Read the model definition and answer for the solid it produces. Units are mm, in the model's axes. A direction names the side the tool comes from. Coordinates: 2 decimals unless noted, no trailing zeros. Write each loop counter-clockwise with the first axis right and the second up, starting at its lowest first coordinate (ties: lowest second). Pieces come first, ordered by that corner, then holes. Notation, with made-up numbers: (87.5, -23.75) - (108.5, -23.75) arc R15 cw to (108.5, -18.75) - close; hole circle Ø4 at (-31, 14). An arc over 180 degrees is marked (long way). Return JSON: item names as keys, results as strings.
Autodesk Inventor part; units mm, degrees
ref_plane "YZ Plane" through (0, 0, 0) normal (1, 0, 0) x (0, 1, 0)
ref_plane "XZ Plane" through (0, 0, 0) normal (0, 1, 0) x (-1, 0, 0)
ref_plane "XY Plane" through (0, 0, 0) normal (0, 0, 1) x (1, 0, 0)
sketch "Sketch1" plane through (0, 0, 0) normal (0, 1, 0) x (-1, 0, 0)
  line L0 (20.0829, 44.2754) -> (-39.9171, 44.2754)
  line L1 (-39.9171, 44.2754) -> (-39.9171, -37.0246)
  line L2 (-39.9171, -37.0246) -> (20.0829, -37.0246)
  line L3 (20.0829, -37.0246) -> (20.0829, 44.2754)
  point P0 (0, 0)
  dimension "d0" = 60
  dimension "d1" = 81.3
extrude "Extrusion1" add sketch "Sketch1" along normal blind 3.175
sketch "Sketch8" plane through (0, 0, 0) normal (0, -1, 0) x (1, 0, 0)
  circle A0 centre (9.4171, 36.2754) radius 1.397
  circle A1 centre (-13.0829, -19.5246) radius 1.397
  circle A2 centre (31.9171, -15.3246) radius 1.397
  line L0 (39.9171, 44.2754) -> (39.9171, -37.0246)
  line L1 (39.9171, -37.0246) -> (-20.0829, -37.0246)
  point P0 (0, 0)
  point P1 (39.9171, 42.2754)
  point P2 (39.9171, -35.0246)
  point P3 (37.9171, -37.0246)
  point P4 (-18.0829, -37.0246)
  dimension "d76" = 8
  dimension "d77" = 21.7
  dimension "d78" = 4.2
  dimension "d79" = 45
  dimension "d80" = 22.5
  dimension "d81" = 51.6
  dimension "d97" = 2.794
extrude "Extrusion6" cut sketch "Sketch8" against normal blind 4
sketch "Sketch9" plane through (0, 0, 0) normal (0, -1, 0) x (1, 0, 0)
  line L0 (39.9171, -37.0246) -> (-20.0829, -37.0246)
  line L1 (-20.0829, -24.3246) -> (39.9171, -24.3246)
  line L2 (39.9171, -24.3246) -> (39.9171, -37.0246)
  line L3 (39.9171, -37.0246) -> (-20.0829, -37.0246)
  line L4 (-20.0829, -37.0246) -> (-20.0829, -24.3246)
  line L5 (39.9171, 44.2754) -> (39.9171, -37.0246)
  line L6 (39.9171, -11.6246) -> (15.7671, -11.6246)
  line L7 (15.7671, -11.6246) -> (15.7671, 7.0444)
  line L8 (15.7671, 7.0444) -> (39.9171, 7.0444)
  line L9 (39.9171, 7.0444) -> (39.9171, -11.6246)
  line L10 (-20.0829, -11.6246) -> (3.0671, -11.6246)
  line L11 (3.0671, -11.6246) -> (3.0671, 7.0444)
  line L12 (3.0671, 7.0444) -> (-20.0829, 7.0444)
  line L13 (-20.0829, 7.0444) -> (-20.0829, -11.6246)
  circle A0 centre (9.4171, 36.2754) radius 1.397 construction
  line L14 (9.4171, 36.2754) -> (9.4171, 34.8784) construction
  line L15 (-20.0829, 44.2754) -> (39.9171, 44.2754) construction
  line L16 (-20.0829, -37.0246) -> (-20.0829, 44.2754)
  line L17 (-20.0829, -37.0246) -> (-20.0829, 44.2754)
  line L18 (-20.0829, 44.2754) -> (3.0671, 44.2754)
  line L19 (3.0671, 44.2754) -> (3.0671, 14.6644)
  line L20 (3.0671, 14.6644) -> (-20.0829, 14.6644)
  line L21 (-20.0829, 14.6644) -> (-20.0829, 44.2754)
  line L22 (-20.0829, 44.2754) -> (39.9171, 44.2754)
  line L23 (15.7671, 14.6644) -> (39.9171, 14.6644)
  line L24 (39.9171, 14.6644) -> (39.9171, 44.2754)
  line L25 (39.9171, 44.2754) -> (15.7671, 44.2754)
  line L26 (15.7671, 44.2754) -> (15.7671, 14.6644)
  line L27 (-20.0829, 14.6644) -> (-8.7773, 14.6644)
  line L28 (-8.7773, 14.6644) -> (-8.7773, 7.0444)
  line L29 (-8.7773, 7.0444) -> (-20.0829, 7.0444)
  line L30 (-20.0829, 7.0444) -> (-20.0829, 14.6644)
  line L31 (39.9171, 14.6644) -> (28.6115, 14.6644)
  line L32 (28.6115, 14.6644) -> (28.6115, 7.0444)
  line L33 (28.6115, 7.0444) -> (39.9171, 7.0444)
  line L34 (39.9171, 7.0444) -> (39.9171, 14.6644)
  line L35 (9.9171, 44.2754) -> (9.9171, -37.0246) construction
  point P0 (0, 0)
  point P1 (3.0671, -2.2901)
  point P2 (39.9171, 7.0444)
  point P3 (-8.7773, 14.6644)
  point P4 (28.6115, 14.6644)
  dimension "d98" = 12.7
  dimension "d99" = 12.7
  dimension "d100" = 12.7
  dimension "d142" = 18.669
  dimension "d143" = 7.62
  dimension "d144" = 37.3888
sketch "Sketch11" plane through (0, 3.175, 0) normal (0, 1, 0) x (1, 0, 0)
  line L0 (3.0671, 11.6246) -> (-20.0829, 11.6246)
  line L1 (-8.7773, 19.2446) -> (-4.3323, 19.2446)
  line L2 (-4.3323, 19.2446) -> (-4.3323, 11.6246)
  line L3 (-4.3323, 11.6246) -> (-8.7773, 11.6246)
  line L4 (-8.7773, 11.6246) -> (-8.7773, 19.2446)
  line L5 (39.9171, 11.6246) -> (15.7671, 11.6246)
  line L6 (24.1665, 19.2446) -> (28.6115, 19.2446)
  line L7 (28.6115, 19.2446) -> (28.6115, 11.6246)
  line L8 (28.6115, 11.6246) -> (24.1665, 11.6246)
  line L9 (24.1665, 11.6246) -> (24.1665, 19.2446)
  line L10 (39.9171, 24.3246) -> (-20.0829, 24.3246) construction
  line L11 (9.9171, 24.3246) -> (9.9171, -44.2754) construction
  line L12 (-20.0829, -44.2754) -> (39.9171, -44.2754) construction
  point P0 (0, 0)
  dimension "d115" = 28.4988
  dimension "d116" = 7.62
  dimension "d117" = 4.445
extrude "Extrusion9" add sketch "Sketch11" against normal blind 15.875
sketch "Sketch12" plane through (28.6115, 3.175, -11.6246) normal (1, 0, 0) x (0, 0, 1)
  line L0 (-7.62, 15.875) -> (0, 15.875)
  line L1 (-7.62, 3.175) -> (-7.62, 15.875)
  point P0 (11.6246, 3.175)
  point P1 (-3.81, 10.795)
  point P2 (7.62, 0)
  dimension "d130" = 5.08
  dimension "d148" = 3.81
hole "Hole1" at (28.6115, -7.62, -15.4346) direction (-1, 0, 0) diameter 3.175 depth 37.3888
pattern_linear "Rectangular Pattern1" count 2 spacing 26.289 along (0, 0, 1) of "Extrusion9", "Hole1"
extrude "Extrusion10" cut sketch "Sketch9" against normal blind 25.4 contours L0 L4 L1 L2 | L6 L7 L8 L5 | L13 L12 L11 L10 | L8 L32 L23 L5 | L16 L20 L28 L12 | L23 L26 L22 L5 | L16 L18 L19 L20
fillet "Fillet2" radius 6.35 4 edges at (3.0671, 1.5875, 44.2754) (15.7671, 1.5875, 44.2754) (-20.0829, 1.5875, -24.3246) (39.9171, 1.5875, -24.3246)
properties part number "TALLER_SkyhopperMount"
(1) A cutting plane is placed at D-D (z = -3). Determine the outline of the cut face in (x, y) (3 decimals).
Answer:
{"outline": "(3.067, 0) - (15.767, 0) - (15.767, 3.175) - (3.067, 3.175) - close"}
(2) Which of the six approach directions +Z, -Z, +X, -X, +Y, -Y give full straight-line access (tool end or side, diameter ignored) to faces 5 (the face through (-6, -1, -11.625)), 6 (the face through (-8.777, -5, -15)), 7 (the face through (24.166, -6, 12)), 8 (the face through (28, -1, -11.625))?
Answer:
{"face 5": "-X, +Y, -Y", "face 6": "+Z, -Z, -X, -Y", "face 7": "+Z, -Z, -Y", "face 8": "+X, +Y, -Y"}
(3) A cutting plane is placed at B-B (x = -3.5). Determine the outline of the cut face in (y, z) (3 decimals).
Answer:
{"outline": "(0, -24.325) - (3.175, -24.325) - (3.175, -11.625) - (0, -11.625) - close; (0, 7.044) - (3.175, 7.044) - (3.175, 14.664) - (0, 14.664) - close"}
(4) Flat-ended cylindrical pins translate along their axes: P1, Ø3, axis at y = -7.62, z = -15.43, coming from the +X side; P2, Ø3.5, axis at x = 31.92, z = -15.32, coming from the +Y side (3 decimals); P3, Ø2.5, axis at y = -8, z = -14.5, coming from the -X side; P4, Ø6, axis at x = -5.5, y = -7.5, coming from the -Z side. Find the tip coordinate at first contact, or state that the pin passes through.
Answer:
{"P1": "through", "P2": "y = 3.175", "P3": "x = -8.78", "P4": "z = -19.24"}
(5) Determine the mould class of faces 1 (the face through (-6.586, -6.212, -16.167)), 2 (the face through (-5, -3, 14.664)), 3 (the face through (-7, -12.7, -15)), 4 (the face through (26.358, -6.212, -16.167)) for opening direction Y: +Y half, -Y half, draft (parallel to the pull), parting line (faces both ways), or undercut.
Answer:
{"face 1": "undercut", "face 2": "draft", "face 3": "-Y half", "face 4": "undercut"}
(6) A cutting plane is placed at A-A (y = -7.62). State how many separate pieces and enclosed holes the cut face has, and give its area (3 significant figures).
Answer:
{"separate pieces": "8", "enclosed holes": "0", "area": "79.0 mm²"}
(7) A cutting plane is placed at C-C (y = -1.5). Determine the outline of the cut face in (x, z), and give its area (3 significant figures).
Answer:
{"outline": "(-8.78, -19.24) - (-4.33, -19.24) - (-4.33, -11.62) - (-8.78, -11.62) - close; (-8.78, 7.04) - (-4.33, 7.04) - (-4.33, 14.66) - (-8.78, 14.66) - close; (24.17, -19.24) - (28.61, -19.24) - (28.61, -11.62) - (24.17, -11.62) - close; (24.17, 7.04) - (28.61, 7.04) - (28.61, 14.66) - (24.17, 14.66) - close", "area": "135 mm²"}
(8) Straight lines are drawn through the part: line 1 (Z direction, x = -7.1, y = -7.62); line 2 (Z direction, x = -5.5, y = 2.75); line 3 (X direction, y = -6, z = -18). For each, find the intervals that lie inside material, in ascending order. Write a range as from..to.
Answer:
{"line 1": "-19.24..-17.02, -13.85..-11.62, 7.04..9.27, 12.44..14.66", "line 2": "-24.32..-11.62, 7.04..14.66", "line 3": "-8.78..-4.33, 24.17..28.61"}
